Geometry check sheet. Reference: the model listing, model coordinates, mm. Face numbers are marked on the shaded views. A direction names the side the tool comes from. Give positions to 0.01 mm unless a question says otherwise; leave off trailing zeros. Loops run counter-clockwise (first coordinate to the right, second up) from the corner with the lowest first, then second, coordinate; pieces in that order, holes last. Notation, with made-up numbers: (78, 11) -> (123, 11) arc R13 cw to (123, 30) -> close; hole circle Ø4 at (-20, -25). An arc over 180 degrees is marked (long way). Write item = value, one per line. Start each with the question number.
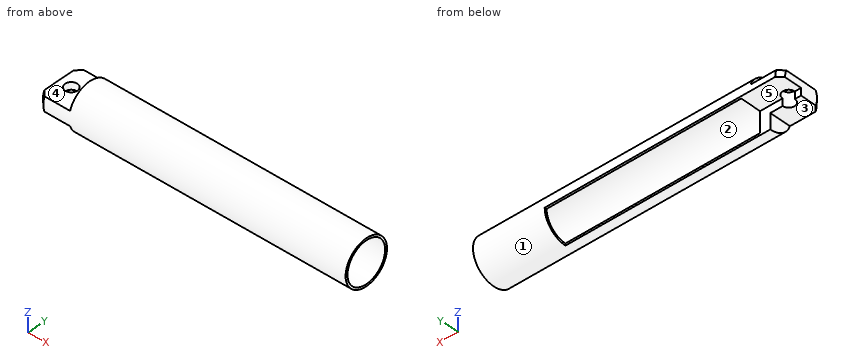
```python
from build123d import *

# Parameters (mm, degrees)
CHANFREIN1_SIZE         = 5
ESQUISSE2_W             = 62.305459945
ESQUISSE2_H             = 30.289532294
ENL_V_MAT_EXTRU_1_DEPTH = 25
ENL_V_MAT_EXTRU_2_REACH = 304.2
ESQUISSE3_R             = 6
ESQUISSE4_W             = 39.235751697
ESQUISSE4_H             = 28.135609998
ENL_V_MAT_EXTRU_3_DEPTH = 230


with BuildPart() as part:
    # Esquisse1 → Révolution1 (revolve)
    with BuildSketch(Plane(origin=(0, 0, 0), x_dir=(1, 0, 0), z_dir=(0, 1, 0)), mode=Mode.PRIVATE) as r_volution1_sk:
        Polygon((0, 0), (0, 22), (300, 22), (300, 20), (40, 20), (40, 0), align=None)
    revolve(r_volution1_sk.sketch.rotate(Axis((0, 0, 0), (1, 0, 0)), 180), axis=Axis((0, 0, 0), (1, 0, 0)))

    # Chanfrein1
    chanfrein1_edges = [part.edges().sort_by_distance(p)[0] for p in [
        (0, 0, -22),
    ]]
    chamfer(chanfrein1_edges, length=CHANFREIN1_SIZE)

    # Esquisse2 → Enlèv. mat.-Extru.1 (cut, symmetric)
    with BuildSketch(Plane(origin=(0, 0, 0), x_dir=(1, 0, 0), z_dir=(0, 1, 0))):
        with Locations((-1.152729972, 22.144766147)):
            Rectangle(ESQUISSE2_W, ESQUISSE2_H)
        with Locations((-1.152729972, -22.144766147)):
            Rectangle(ESQUISSE2_W, ESQUISSE2_H)
    extrude(amount=ENL_V_MAT_EXTRU_1_DEPTH, both=True, mode=Mode.SUBTRACT)

    # Esquisse3 → Enlèv. mat.-Extru.2 (cut, up to next)
    with BuildSketch(Plane(origin=(0, 0, -7), x_dir=(-1, 0, 0), z_dir=(0, 0, -1)), mode=Mode.PRIVATE) as enl_v_mat_extru_2_sk1:
        with Locations((-12, 0)):
            Circle(ESQUISSE3_R)
    enl_v_mat_extru_2_tool1 = extrude(enl_v_mat_extru_2_sk1.sketch, amount=-ENL_V_MAT_EXTRU_2_REACH, mode=Mode.PRIVATE) & part.part
    add(enl_v_mat_extru_2_tool1.solids().sort_by_distance((12, 0, -7))[0], mode=Mode.SUBTRACT)

    # Esquisse4 → Enlèv. mat.-Extru.3 (cut)
    with BuildSketch(Plane(origin=(0, 0, 0), x_dir=(0, 0, -1), z_dir=(1, 0, 0))):
        with Locations((19.617875849, 14.067804999)):
            Rectangle(ESQUISSE4_W, ESQUISSE4_H)
    extrude(amount=ENL_V_MAT_EXTRU_3_DEPTH, mode=Mode.SUBTRACT)


solid = part.part
```
1) Depth check by flat-ended pin: pin 1 Ø3 at (x, z) = (2.5, -3.5) entering from +Y; pin 2 Ø1.5 at (x, y) = (140, 6.5) entering from -Z; pin 3 Ø1 at (x, y) = (61, 16.5) entering from +Z. Enter the tip coordinate at first touch or a pass-through.
2) Thickness scan on line 1 (X direction, y = 0, z = 1.25); line 2 (Y direction, x = 236, z = 0); line 3 (X direction, y = 19.5, z = 8). Record the ranges inside material, lowest first.
3) Section check B-B (z = -12.5). Enter the section's corners in (x, y), plus the area to 3 significant figures.
4) Section check C-C (x = 247). Enter the section's corners in (y, z).
5) Section check D-D (z = 15.5). Enter the section's corners in (x, y), plus the area to 3 significant figures.
6) Draft check along Y on the marked faces 1, 2 and 3. Enter one of: released by +Y, released by -Y, zero draft, split by the parting line, or undercut.
7) Section check A-A (x = 12). Enter the section's corners in (y, z), plus the area to 3 significant figures.
8) Tool access check on the marked faces 4 and 5. Record the directions out of +Z, -Z, +X, -X, +Y, -Y that give a thin tool (end or side, any length) a straight path to the whole face; none if there is none.
Check result:
q1.pin_1 = 0
q1.pin_2 = 18.64
q1.pin_3 = 15.1
q2.line_1 = 0 to 6, 18 to 40
q2.line_2 = -22 to -20, 20 to 22
q2.line_3 = 30 to 300
q3.outline = (30, -18.1) -> (300, -18.1) -> (300, -15.61) -> (40, -15.61) -> (40, 0) -> (30, 0) -> close; (230, 15.61) -> (300, 15.61) -> (300, 18.1) -> (230, 18.1) -> close
q3.area = 1,000 mm2
q4.outline = circle Ø44 at (0, 0); hole circle Ø40 at (0, 0)
q5.outline = (30, -15.61) -> (300, -15.61) -> (300, -12.64) -> (40, -12.64) -> (40, 12.64) -> (300, 12.64) -> (300, 15.61) -> (30, 15.61) -> close
q5.area = 1,860 mm2
q6.face_1 = split by the parting line
q6.face_2 = undercut
q6.face_3 = zero draft
q7.outline = (-20.86, -7) -> (-6, -7) -> (-6, 7) -> (-20.86, 7) arc R22 ccw to start; (6, 0) -> (22, 0) arc R22 ccw to (20.86, 7) -> (6, 7) -> close
q7.area = 328 mm2
q8.face_4 = +Z, -X, +Y, -Y
q8.face_5 = -Z, -X, +Y
